Geometry check sheet. Reference: the model listing, model coordinates, mm. Round coordinates to 2 decimals unless told otherwise and drop trailing zeros. Order: outer loops, then holes, each group sorted by start corner. A loop starts at its lowest first (then second) coordinate and runs counter-clockwise, first axis right, second up.
(1) Cross-section at D-D on x = -62. Enter the section's corners in (y, z), and give its area (3 significant figures).
(2) Cross-section at C-C on y = 8.5. Count the separate pieces of the cut face and the enclosed holes in it, and give its area (3 significant figures).
(3) Thickness scan on L1, parallel to X at y = 7.25, z = -25; L2, parallel to X at y = 7.75, z = -56; L3, parallel to Z at x = -16.5, y = 8. Record the ranges inside material, lowest first.
(4) Cross-section at B-B on z = -17. Enter the section's corners in (x, y), and give its area (3 significant figures).
(5) Gauge pin test, flat ends, axial feed: P1, Ø3, axis at x = 21, y = 7, coming from the +Z side; P2, Ø5, axis at y = 3, z = -22.5, coming from the -X side; P3, Ø5, axis at x = 16, y = 6, coming from the -Z side. Record the tip position at first contact, or that the pin passes through.
(6) Cross-section at A-A on x = -17. Enter the section's corners in (y, z).
from build123d import *

# Parameters (mm, degrees)
BOSS_EXTRUDE1_DEPTH = 10
BOSS_EXTRUDE2_DEPTH = 10
SKETCH2_R           = 1.5
CUT_EXTRUDE1_DEPTH  = 147.372811683


with BuildPart() as part:
    # Sketch1 → Boss-Extrude1 (new body)
    with BuildSketch(Plane(origin=(0, 0, 0), x_dir=(1, 0, 0), z_dir=(0, 1, 0))):
        Polygon((-115, -10), (-10, -10), (-10, -90), (10, -90), (10, -10), (115, -10), (115, 10), (10, 10), (10, 90), (-10, 90), (-10, 10), (-115, 10), align=None)
    extrude(amount=BOSS_EXTRUDE1_DEPTH)

    # Sketch3 → Boss-Extrude2 (add)
    with BuildSketch(Plane(origin=(0, 0, 0), x_dir=(1, 0, 0), z_dir=(0, 1, 0))):
        Polygon((0, -56.568542495), (56.568542495, 0), (0, 56.568542495), (-56.568542495, 0), align=None)
        Polygon((0, -42.426406871), (42.426406871, 0), (0, 42.426406871), (-42.426406871, 0), align=None, mode=Mode.SUBTRACT)
    extrude(amount=BOSS_EXTRUDE2_DEPTH)

    # Sketch2 → Cut-Extrude1 (cut, through all)
    with BuildSketch(Plane(origin=(0, 10, 0), x_dir=(1, 0, 0), z_dir=(0, 1, 0))):
        with Locations(Location((0, 0, 0), (0, 0, 270))):
            Circle(SKETCH2_R)
        with Locations(Location((36, 0, 0), (0, 0, 270))):
            Circle(SKETCH2_R)
        with Locations(Location((72, 0, 0), (0, 0, 270))):
            Circle(SKETCH2_R)
        with Locations(Location((108, 0, 0), (0, 0, 270))):
            Circle(SKETCH2_R)
        with Locations(Location((0, 28, 0), (0, 0, 270))):
            Circle(SKETCH2_R)
        with Locations(Location((-36, 0, 0), (0, 0, 270))):
            Circle(SKETCH2_R)
        with Locations(Location((-72, 0, 0), (0, 0, 270))):
            Circle(SKETCH2_R)
        with Locations(Location((-108, 0, 0), (0, 0, 270))):
            Circle(SKETCH2_R)
        with Locations(Location((0, 56, 0), (0, 0, 270))):
            Circle(SKETCH2_R)
        with Locations(Location((0, 84, 0), (0, 0, 270))):
            Circle(SKETCH2_R)
        with Locations(Location((0, -28, 0), (0, 0, 270))):
            Circle(SKETCH2_R)
        with Locations(Location((0, -56, 0), (0, 0, 270))):
            Circle(SKETCH2_R)
        with Locations(Location((0, -84, 0), (0, 0, 270))):
            Circle(SKETCH2_R)
    extrude(amount=-CUT_EXTRUDE1_DEPTH, mode=Mode.SUBTRACT)


solid = part.part
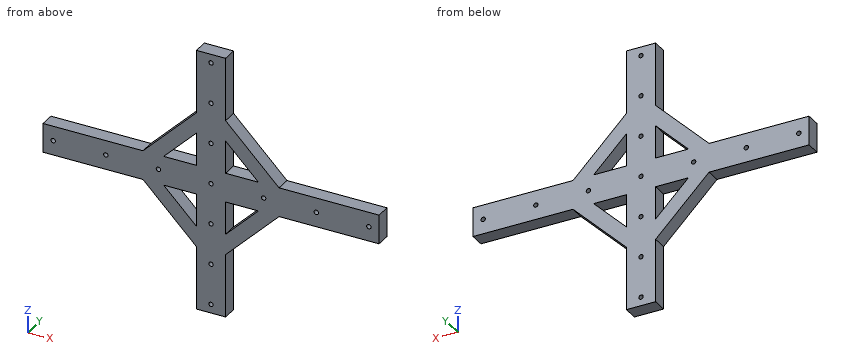
Found:
1. outline: (0, -10) - (10, -10) - (10, 10) - (0, 10) - close
1. area: 200 mm2
2. separate pieces: 1
2. enclosed holes: 17
2. area: 9,380 mm2
3. L1: x = -31.57 to -17.43, -10 to 10, 17.43 to 31.57
3. L2: x = -10 to -1.5, 1.5 to 10
3. L3: z = -40.07 to -25.93, -10 to 10, 25.93 to 40.07
4. outline: (-39.57, 0) - (-25.43, 0) - (-25.43, 10) - (-39.57, 10) - close; (-10, 0) - (10, 0) - (10, 10) - (-10, 10) - close; (25.43, 0) - (39.57, 0) - (39.57, 10) - (25.43, 10) - close
4. area: 483 mm2
5. P1: stops at z = 37.07
5. P2: stops at x = -36.57
5. P3: stops at z = -43.07
6. outline: (0, -39.57) - (10, -39.57) - (10, -25.43) - (0, -25.43) - close; (0, -10) - (10, -10) - (10, 10) - (0, 10) - close; (0, 25.43) - (10, 25.43) - (10, 39.57) - (0, 39.57) - close
